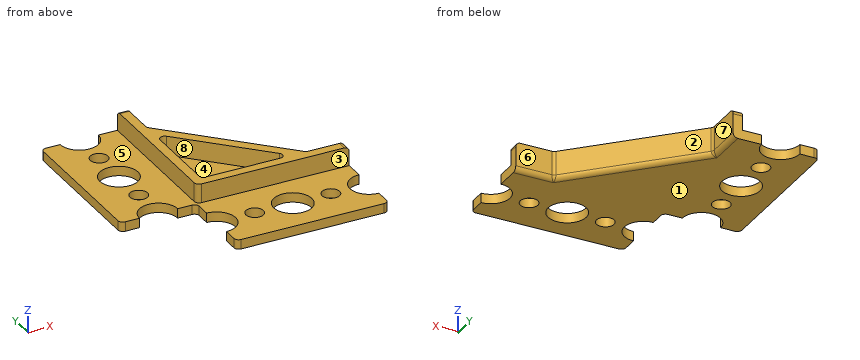
Autodesk Inventor part; units mm, degrees
ref_plane "РабПлоскость1" through (0, 0, 2) normal (0, 0, 1) x (1, 0, 0)
ref_plane "YZ Plane" through (0, 0, 0) normal (1, 0, 0) x (0, 1, 0)
ref_plane "XZ Plane" through (0, 0, 0) normal (0, 1, 0) x (-1, 0, 0)
sketch "Эскиз1" plane through (0, 0, 0) normal (0, 0, 1) x (1, 0, 0)
  line L0 (0, 16) -> (0, 48)
  line L1 (0, 48) -> (4, 48)
  arc A0 (4, 48) -> (12, 48) centre (8, 48) ccw
  line L2 (12, 48) -> (18, 48)
  line L3 (18, 48) -> (18, 40)
  line L4 (18, 40) -> (40, 18)
  line L5 (40, 18) -> (48, 18)
  line L6 (48, 18) -> (48, 12)
  arc A1 (48, 12) -> (48, 4) centre (48, 8) ccw
  line L7 (48, 4) -> (48, 0)
  line L8 (48, 0) -> (16, 0)
  line L9 (16, 0) -> (16, 4)
  arc A2 (16, 4) -> (16, 12) centre (16, 8) ccw
  line L10 (16, 12) -> (16, 16)
  line L11 (16, 16) -> (12, 16)
  arc A3 (12, 16) -> (4, 16) centre (8, 16) ccw
  line L12 (0, 16) -> (4, 16)
  circle A4 centre (8, 24) radius 1.85
  circle A5 centre (8, 32) radius 4
  circle A6 centre (8, 40) radius 1.85
  circle A7 centre (40, 8) radius 1.85
  circle A8 centre (32, 8) radius 4
  circle A9 centre (24, 8) radius 1.85
extrude "Выдавливание1" add sketch "Эскиз1" along normal blind 2
fillet "Сопряжение1" radius 1 8 edges at (0, 48, 1) (18, 44, 0) (29, 29, 0) (44, 18, 0) (48, 0, 1) (16, 0, 1) (16, 16, 1) (0, 16, 1)
ref_plane "РабПлоскость1" through (0, 0, 2) normal (0, 0, 1) x (1, 0, 0)
sketch "Эскиз2" plane through (0, 0, 2) normal (0, 0, 1) x (1, 0, 0)
  line L0 (16, 16) -> (16, 48)
  line L1 (16, 48) -> (18, 48)
  line L2 (18, 48) -> (18, 40)
  line L3 (18, 40) -> (40, 18)
  line L4 (40, 18) -> (48, 18)
  line L5 (48, 18) -> (48, 16)
  line L6 (16, 16) -> (48, 16)
  line L7 (18, 18) -> (18, 37)
  line L8 (18, 37) -> (37, 18)
  line L9 (18, 18) -> (37, 18)
extrude "Выдавливание2" add sketch "Эскиз2" along normal blind 4
fillet "Сопряжение2" radius 1 8 edges at (37, 18, 4) (18, 37, 4) (18, 18, 4) (16, 16, 4) (48, 17, 6) (17, 48, 6) (17.7071, 39.8787, 0.2929) (39.8787, 17.7071, 0.2929)
Check sheet for the modelled part. Datum: model origin and axes. Units: mm. Face numbers are marked on the shaded views. A direction names the side the tool comes from. Give positions to 0.01 mm unless a question says otherwise; leave off trailing zeros. Write each loop counter-clockwise with the first axis right and the second up, starting at its lowest first coordinate (ties: lowest second). Pieces come first, ordered by that corner, then holes.
Item 1: Gauge pin test, flat ends, axial feed: pin 1 (2.5 mm diameter, centred on y = 45, z = 3, fed in from +X); pin 2 (1.5 mm diameter, centred on x = 29, z = 4, fed in from +Y); pin 3 (0.6 mm diameter, centred on x = 2, z = 1.5, fed in from -Y). Record the tip position at first contact, or that the pin passes through.
Item 2: Cross-section at A-A (y = 11). Enter the section's corners in (x, z).
Item 3: Access from +Z, -Z, +X, -X, +Y, -Y to the whole of each face (thin tool, end or side, straight path). Record for the marked faces 1, 2, 3, 4 and 5.
Item 4: Draft check along X on the marked faces 6, 7 and 8. Enter one of: released by +X, released by -X, zero draft, split by the parting line, or undercut.
Item 5: Cross-section at C-C (x = 7.5). Enter the section's corners in (y, z).
Item 6: Cross-section at B-B (z = 3). Enter the section's corners in (x, y).
Item 7: Scan lines: L1, parallel to Y at x = 9, z = 1; L2, parallel to X at y = 9.5, z = 1; L3, parallel to Z at x = 28, y = 12. Record each from-to range of solid material in increasing order.
Report:
1. pin 1: stops at x = 18
1. pin 2: stops at y = 29.75
1. pin 3: stops at y = 16
2. outline: (18.65, 0) - (29.35, 0) - (29.35, 2) - (18.65, 2) - close; (34.65, 0) - (45.35, 0) - (45.35, 2) - (34.65, 2) - close
3. face 1: -Z, +X, -X, +Y, -Y
3. face 2: +Z, -Z, +X, +Y
3. face 3: +Z, +X, -X, -Y
3. face 4: +Z
3. face 5: +Z, -X, -Y
4. face 6: zero draft
4. face 7: released by +X
4. face 8: undercut
5. outline: (19.97, 0) - (22.22, 0) - (22.22, 2) - (19.97, 2) - close; (25.78, 0) - (28.03, 0) - (28.03, 2) - (25.78, 2) - close; (35.97, 0) - (38.22, 0) - (38.22, 2) - (35.97, 2) - close; (41.78, 0) - (44.03, 0) - (44.03, 2) - (41.78, 2) - close
6. outline: (16, 17) arc R1 ccw to (17, 16) - (48, 16) - (48, 18) - (40.41, 18) arc R1 cw to (39.71, 18.29) - (18.29, 39.71) arc R1 cw to (18, 40.41) - (18, 48) - (16, 48) - close; hole (18, 19) arc R1 ccw to (19, 18) - (34.59, 18) arc R1 ccw to (35.29, 19.71) - (19.71, 35.29) arc R1 ccw to (18, 34.59) - close
7. L1: y = 19.87 to 22.44, 25.56 to 28.13, 35.87 to 38.44, 41.56 to 44.13
7. L2: x = 19.71 to 22.92, 25.08 to 28.29, 35.71 to 38.92, 41.08 to 44.29
7. L3: z = 0 to 2
